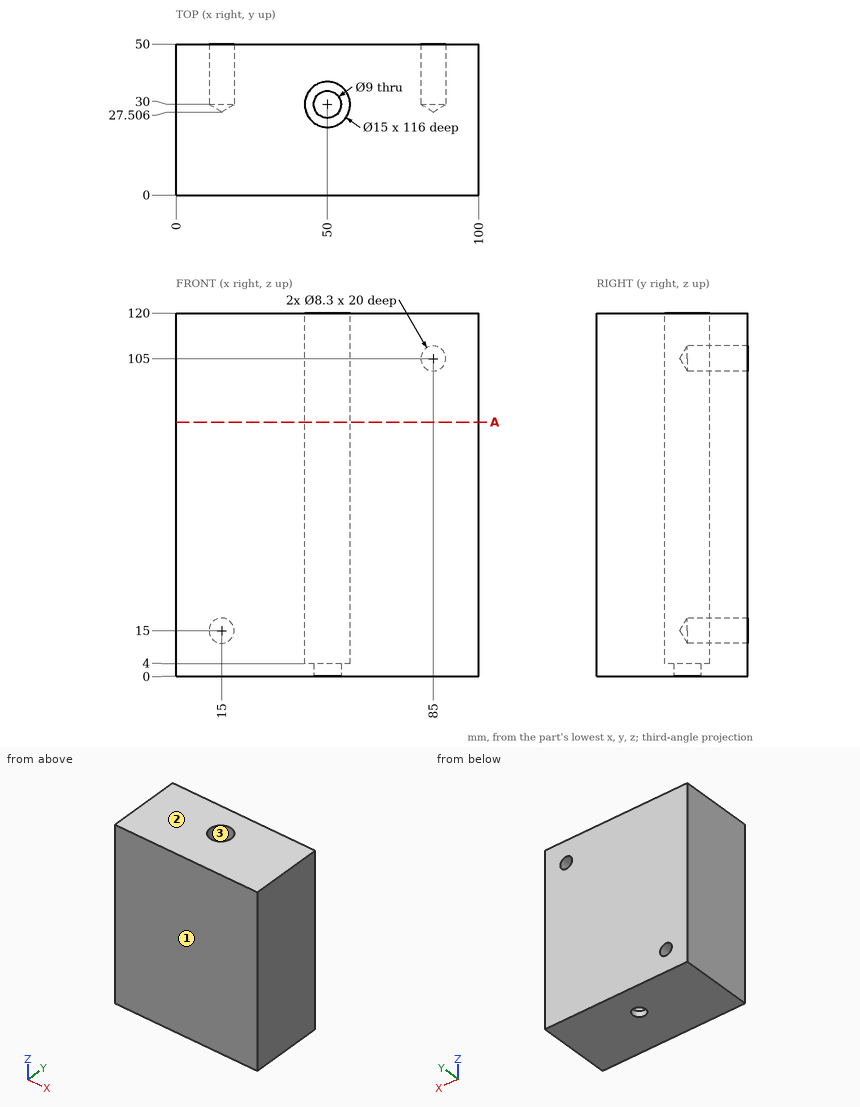
Drawing for the job (mm, zero at the part's lowest x, y, z). Give positions to 0.01 mm unless a question says otherwise; leave off trailing zeros. Write each loop counter-clockwise with the first axis right and the second up, starting at its lowest first coordinate (ties: lowest second). Pieces come first, ordered by that corner, then holes. Notation, with made-up numbers: M 71,0 L 108,0 A24 ccw 108,23 Z; hole C -2,-28.5 d1. An arc over 180 degrees is marked long. Return JSON: item names as keys, results as strings. Group by question number.
(1) Flat gauge pins, fed straight in: pin 1 Ø1.5 at (y, z) = (19.5, 73) entering from -X; pin 2 Ø7.5 at (x, y) = (48.5, 28.5) entering from +Z; pin 3 Ø5 at (x, z) = (15, 15) entering from +Y; pin 4 Ø6.5 at (x, z) = (85, 105) entering from +Y. Where does each tip first touch, or does it go through?
(2) Band-saw the part on A-A (z = 84). Give the cut face in (x, y).
(3) Drill centre lines: L1, parallel to X at y = 36, z = 105; L2, parallel to Z at x = 15, y = 44.25; L3, parallel to Z at x = 85, y = 44.25. Where is each one in solid material? Low to high. Write a range as [from, to].
(4) Mould opens along Y. For the marked faces 1, 2 and 3 say: pulls with the +Y half, pulls with the -Y half, needs draft (parallel to the pull), parting line crosses it, or undercut.
Entries:
{
 "1": {"pin 1": "stops at x = 0", "pin 2": "stops at z = 4", "pin 3": "stops at y = 29.01", "pin 4": "stops at y = 29.46"},
 "2": {"outline": "M 0,0 L 100,0 L 100,50 L 0,50 Z; hole C 50,30 d15"},
 "3": {"L1": "x = [0, 45.5], [54.5, 80.85], [89.15, 100]", "L2": "z = [0, 10.85], [19.15, 120]", "L3": "z = [0, 100.85], [109.15, 120]"},
 "4": {"face 1": "pulls with the -Y half", "face 2": "needs draft", "face 3": "undercut"}
}
